Design review of the part built by this model. Coordinates are the model's own, in mm. Face numbers are marked on the shaded views. A direction names the side the tool comes from. Round coordinates to 2 decimals unless told otherwise and drop trailing zeros. Order: outer loops, then holes, each group sorted by start corner. A loop starts at its lowest first (then second) coordinate and runs counter-clockwise, first axis right, second up. Notation, with made-up numbers: (-29.5, 49) - (-17.5, 49) arc R19 cw to (-17.5, 86) - close; hole circle Ø4 at (-5, 51). An arc over 180 degrees is marked (long way). Use CSV: the item, a comma, the result in double quotes.
from build123d import *
from OCP.BRepFilletAPI import BRepFilletAPI_MakeChamfer

# Parameters (mm, degrees)
SKETCH1_W          = 20.2
SKETCH1_H          = 40.2
EXTRUDE1_DEPTH     = 25.4
SKETCH2_W          = 20.2
SKETCH2_H          = 40.2
EXTRUDE2_DEPTH     = 2.38125
SKETCH3_W          = 20.2
SKETCH3_H          = 40.2
EXTRUDE3_DEPTH     = 4.445
EXTRUDE4_DEPTH     = 2.38125
SKETCH5_R          = 7.62
EXTRUDE5_DEPTH     = 3.4925
SKETCH7_W          = 3.5
SKETCH7_H          = 1
EXTRUDE6_DEPTH     = 0.635
SKETCH8_R          = 2.778125
EXTRUDE7_DEPTH     = 3.175
CHAMFER2_SIZE      = 2.54
CHAMFER2_SIZE2     = 1.466469684
FILLET1_R          = 1.016
FILLET2_R          = 1.524
SKETCH9_W          = 6.35
SKETCH9_H          = 2.54
EXTRUDE8_DEPTH     = 2.38125
SKETCH10_W         = 5.08
SKETCH10_H         = 1.27
CUT_EXTRUDE1_DEPTH = 2.38125
CHAMFER3_SIZE      = 0.3
SKETCH11_R         = 3.778125
CUT_EXTRUDE2_DEPTH = 3.175
SKETCH12_R         = 1.15
CUT_EXTRUDE3_DEPTH = 3
CUT_EXTRUDE4_START = -1.5
SKETCH13_R         = 7.62
SKETCH13_R_2       = 5
CUT_EXTRUDE4_DEPTH = 1.5


with BuildPart() as part:
    # Sketch1 → Extrude1 (new body)
    with BuildSketch(Plane(origin=(0, 0, 0), x_dir=(1, 0, 0), z_dir=(0, 1, 0))):
        with Locations((0, -9.94)):
            Rectangle(SKETCH1_W, SKETCH1_H)
    extrude(amount=EXTRUDE1_DEPTH)

    # Sketch2 → Extrude2 (add)
    with BuildSketch(Plane(origin=(0, 25.4, 0), x_dir=(-1, 0, 0), z_dir=(0, 1, 0))):
        with Locations((0, 9.94)):
            Rectangle(SKETCH2_W, SKETCH2_H)
        with BuildLine():
            ThreePointArc((6.731, -15.51418631), (5.08, -11.7094), (3.429, -15.51418631))
            Line((3.429, -15.51418631), (3.429, -16.4846))
            Line((3.429, -16.4846), (-3.429, -16.4846))
            Line((-3.429, -16.4846), (-3.429, -15.51418631))
            ThreePointArc((-3.429, -15.51418631), (-5.08, -11.7094), (-6.731, -15.51418631))
            Line((-6.731, -15.51418631), (-6.731, -16.4846))
            Line((-6.731, -16.4846), (-10.1, -16.4846))
            Line((-10.1, -16.4846), (-10.1, -10.16))
            Line((-10.1, -10.16), (10.1, -10.16))
            Line((10.1, -10.16), (10.1, -16.4846))
            Line((10.1, -16.4846), (6.731, -16.4846))
            Line((6.731, -16.4846), (6.731, -15.51418631))
        make_face()
        with BuildLine():
            ThreePointArc((-6.731, 35.83418631), (-5.08, 32.0294), (-3.429, 35.83418631))
            Line((-3.429, 35.83418631), (-3.429, 36.3646))
            Line((-3.429, 36.3646), (3.429, 36.3646))
            Line((3.429, 36.3646), (3.429, 35.83418631))
            ThreePointArc((3.429, 35.83418631), (5.08, 32.0294), (6.731, 35.83418631))
            Line((6.731, 35.83418631), (6.731, 36.3646))
            Line((6.731, 36.3646), (10.1, 36.3646))
            Line((10.1, 36.3646), (10.1, 30.04))
            Line((10.1, 30.04), (-10.1, 30.04))
            Line((-10.1, 30.04), (-10.1, 36.3646))
            Line((-10.1, 36.3646), (-6.731, 36.3646))
            Line((-6.731, 36.3646), (-6.731, 35.83418631))
        make_face()
    extrude(amount=EXTRUDE2_DEPTH)

    # Sketch3 → Extrude3 (add)
    with BuildSketch(Plane(origin=(0, 27.78125, 0), x_dir=(-1, 0, 0), z_dir=(0, 1, 0))):
        with Locations((0, 9.94)):
            Rectangle(SKETCH3_W, SKETCH3_H)
    extrude(amount=EXTRUDE3_DEPTH)

    # Sketch4 → Extrude4 (add)
    with BuildSketch(Plane(origin=(0, 32.22625, 0), x_dir=(-1, 0, 0), z_dir=(0, 1, 0))):
        with BuildLine():
            Line((9.652, 2.228840954), (9.652, 23.69))
            Line((9.652, 23.69), (4.655896906, 23.69))
            ThreePointArc((4.655896906, 23.69), (0, 26.738), (-4.655896906, 23.69))
            Line((-4.655896906, 23.69), (-9.652, 23.69))
            Line((-9.652, 23.69), (-9.652, 2.228840954))
            ThreePointArc((-9.652, 2.228840954), (0, -9.906), (9.652, 2.228840954))
        make_face()
    extrude(amount=EXTRUDE4_DEPTH)

    # Sketch5 → Extrude5 (add)
    with BuildSketch(Plane(origin=(0, 34.6075, 0), x_dir=(-1, 0, 0), z_dir=(0, 1, 0))):
        with Locations(Location((0, 0, 0), (0, 0, 270))):
            Circle(SKETCH5_R)
    extrude(amount=EXTRUDE5_DEPTH)

    # Sketch7 → Extrude6 (add, symmetric)
    with BuildSketch(Plane(origin=(0, 0, 0), x_dir=(0, 0, -1), z_dir=(1, 0, 0))):
        with Locations((11.91, 28.28125)):
            Rectangle(SKETCH7_W, SKETCH7_H)
    extrude6 = extrude(amount=EXTRUDE6_DEPTH, both=True)

    # Mirror1: Extrude6 across plane
    add(extrude6.mirror(Plane.XY.offset(9.72)))

    # Sketch8 → Extrude7 (add)
    with BuildSketch(Plane(origin=(0, 38.1, 0), x_dir=(-1, 0, 0), z_dir=(0, 1, 0))):
        with Locations(Location((0, 0, 0), (0, 0, 270))):
            Circle(SKETCH8_R)
    extrude(amount=EXTRUDE7_DEPTH)

    # Chamfer2: one chamfer whose edges measure the first distance from different faces: ONE call of the kernel's chamfer builder (chamfer() names one face for all edges)
    chamfer2_edges_1 = [part.edges().sort_by_distance(p)[0] for p in [
        (0, 0, -10.16),
    ]]
    chamfer2_side_1 = [part.faces().sort_by_distance(p)[0] for p in [
        (0, 12.7, -10.16),
    ]]
    chamfer2_edges_2 = [part.edges().sort_by_distance(p)[0] for p in [
        (0, 0, 30.04),
    ]]
    chamfer2_side_2 = [part.faces().sort_by_distance(p)[0] for p in [
        (0, 12.7, 30.04),
    ]]
    chamfer2 = BRepFilletAPI_MakeChamfer(part.part.solid().wrapped)
    for e in chamfer2_edges_1:
        chamfer2.Add(CHAMFER2_SIZE, CHAMFER2_SIZE2, e.wrapped, chamfer2_side_1[0].wrapped)  # the first distance lies on this face
    for e in chamfer2_edges_2:
        chamfer2.Add(CHAMFER2_SIZE, CHAMFER2_SIZE2, e.wrapped, chamfer2_side_2[0].wrapped)  # the first distance lies on this face
    add(Compound.cast(chamfer2.Shape()), mode=Mode.REPLACE)

    # Fillet1
    fillet1_edges = [part.edges().sort_by_distance(p)[0] for p in [
        (-10.1, 30.00375, -10.16),
        (10.1, 30.00375, -10.16),
        (10.1, 30.00375, 30.04),
        (10.1, 0, 9.94),
        (10.1, 1.27, -9.426765158),
        (10.1, 13.97, -10.16),
        (0, 0, -8.693530316),
        (0, 2.54, -10.16),
        (-10.1, 13.97, -10.16),
        (-10.1, 1.27, -9.426765158),
        (10.1, 13.97, 30.04),
        (10.1, 1.27, 29.306765158),
        (0, 2.54, 30.04),
        (-10.1, 0, 9.94),
        (0, 0, 28.573530316),
        (-10.1, 1.27, 29.306765158),
        (-10.1, 13.97, 30.04),
        (-10.1, 30.00375, 30.04),
    ]]
    fillet(fillet1_edges, radius=FILLET1_R)

    # Fillet2
    fillet2_edges = [part.edges().sort_by_distance(p)[0] for p in [
        (-10.1, 26.590625, 36.3646),
        (10.1, 26.590625, 36.3646),
        (-10.1, 26.590625, -16.4846),
        (10.1, 26.590625, -16.4846),
    ]]
    fillet(fillet2_edges, radius=FILLET2_R)

    # Sketch9 → Extrude8 (add)
    with BuildSketch(Plane(origin=(0, 0, -10.16), x_dir=(-1, 0, 0), z_dir=(0, 0, -1))):
        with Locations((0, 4.318)):
            Rectangle(SKETCH9_W, SKETCH9_H)
    extrude(amount=EXTRUDE8_DEPTH)

    # Sketch10 → Cut-Extrude1 (cut)
    with BuildSketch(Plane(origin=(0, 0, -12.54125), x_dir=(-1, 0, 0), z_dir=(0, 0, -1))):
        with Locations((0, 4.318)):
            Rectangle(SKETCH10_W, SKETCH10_H)
    extrude(amount=-CUT_EXTRUDE1_DEPTH, mode=Mode.SUBTRACT)

    # Chamfer3
    chamfer3_edges = [part.edges().sort_by_distance(p)[0] for p in [
        (0, 41.275, 2.778125),
    ]]
    chamfer(chamfer3_edges, length=CHAMFER3_SIZE)

    # Sketch11 → Cut-Extrude2 (cut)
    with BuildSketch(Plane(origin=(0, 41.275, 0), x_dir=(1, 0, 0), z_dir=(0, 1, 0))):
        Circle(SKETCH11_R)
        Polygon((0, -2.778125), (-0.336512839, -2.556068783), (-0.71903166, -2.683462686), (-0.986605724, -2.38187692), (-1.3890625, -2.405926825), (-1.569463059, -2.04536408), (-1.964431026, -1.964431026), (-2.04536408, -1.569463059), (-2.405926825, -1.3890625), (-2.38187692, -0.986605724), (-2.683462686, -0.71903166), (-2.556068783, -0.336512839), (-2.778125, 0), (-2.556068783, 0.336512839), (-2.683462686, 0.71903166), (-2.38187692, 0.986605724), (-2.405926825, 1.3890625), (-2.04536408, 1.569463059), (-1.964431026, 1.964431026), (-1.569463059, 2.04536408), (-1.3890625, 2.405926825), (-0.986605724, 2.38187692), (-0.71903166, 2.683462686), (-0.336512839, 2.556068783), (0, 2.778125), (0.336512839, 2.556068783), (0.71903166, 2.683462686), (0.986605724, 2.38187692), (1.3890625, 2.405926825), (1.569463059, 2.04536408), (1.964431026, 1.964431026), (2.04536408, 1.569463059), (2.405926825, 1.3890625), (2.38187692, 0.986605724), (2.683462686, 0.71903166), (2.556068783, 0.336512839), (2.778125, 0), (2.556068783, -0.336512839), (2.683462686, -0.71903166), (2.38187692, -0.986605724), (2.405926825, -1.3890625), (2.04536408, -1.569463059), (1.964431026, -1.964431026), (1.569463059, -2.04536408), (1.3890625, -2.405926825), (0.986605724, -2.38187692), (0.71903166, -2.683462686), (0.336512839, -2.556068783), align=None, mode=Mode.SUBTRACT)
    extrude(amount=-CUT_EXTRUDE2_DEPTH, mode=Mode.SUBTRACT)

    # Sketch12 → Cut-Extrude3 (cut)
    with BuildSketch(Plane(origin=(0, 41.275, 0), x_dir=(1, 0, 0), z_dir=(0, 1, 0))):
        with Locations(Location((0, 0, 0), (0, 0, 270))):
            Circle(SKETCH12_R)
    extrude(amount=-CUT_EXTRUDE3_DEPTH, mode=Mode.SUBTRACT)

    # Sketch13 → Cut-Extrude4 (cut)
    with BuildSketch(Plane(origin=(0, 38.1, 0), x_dir=(1, 0, 0), z_dir=(0, 1, 0)).offset(CUT_EXTRUDE4_START)):
        with Locations(Location((0, 0, 0), (0, 0, 90))):
            Circle(SKETCH13_R)
        with Locations(Location((0, 0, 0), (0, 0, 270))):
            Circle(SKETCH13_R_2, mode=Mode.SUBTRACT)
    extrude(amount=CUT_EXTRUDE4_DEPTH, mode=Mode.SUBTRACT)


solid = part.part
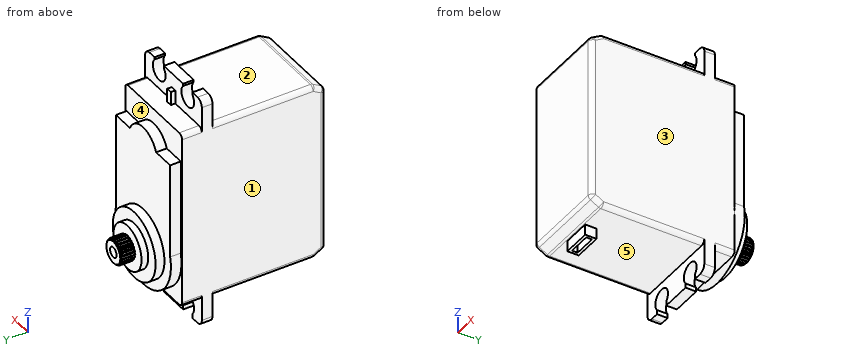
1) We need section D-D (y = 34). Give the boundary of the cut face in (x, z), then the cut area to 3 significant figures.
Data:
outline,"(-9.65, 2.23) arc R9.91 ccw (long way) to (9.65, 2.23) - (9.65, 23.69) - (4.66, 23.69) arc R5.08 ccw to (-4.66, 23.69) - (-9.65, 23.69) - close"
area,"633 mm2"
2) The part is to be moulded in two halves that separate along Y. For the marked faces 3, 4 and 5, say which applies: +Y half, -Y half, draft (parallel to the pull), parting line (faces both ways), or undercut.
Data:
face 3,"draft"
face 4,"+Y half"
face 5,"undercut"
3) We need section B-B (y = 26.5). Give the boundary of the cut face in (x, z).
Data:
outline,"(-10.1, -14.96) arc R1.52 ccw to (-8.58, -16.48) - (-6.73, -16.48) - (-6.73, -15.51) arc R2.26 cw (long way) to (-3.43, -15.51) - (-3.43, -16.48) - (3.43, -16.48) - (3.43, -15.51) arc R2.26 cw (long way) to (6.73, -15.51) - (6.73, -16.48) - (8.58, -16.48) arc R1.52 ccw to (10.1, -14.96) - (10.1, 34.84) arc R1.52 ccw to (8.58, 36.36) - (6.73, 36.36) - (6.73, 35.83) arc R2.26 cw (long way) to (3.43, 35.83) - (3.43, 36.36) - (-3.43, 36.36) - (-3.43, 35.83) arc R2.26 cw (long way) to (-6.73, 35.83) - (-6.73, 36.36) - (-8.58, 36.36) arc R1.52 ccw to (-10.1, 34.84) - close"
4) To check wall thickness, follow L1, parallel to X at y = 26.1, z = 34.29; L2, parallel to Y at x = -0.5, z = -10.5; L3, parallel to Z at x = -6, y = 28.5. State the ranges of each line that lie inside material, in increasing order. Write a range as from..to.
Data:
L1,"x = -10.1..-7.34, -2.82..2.82, 7.34..10.1"
L2,"y = 3.05..3.68, 4.95..5.59, 25.4..28.78"
L3,"z = -10.16..30.04"
5) Insertion check: pin 1 Ø2.5 at (y, z) = (34, 9.5) entering from -X; pin 2 Ø2 at (x, y) = (-4, 21) entering from +Z; pin 3 Ø1 at (x, y) = (5, 26.5) entering from -Z. Each pin has a flat end and moves straight along its axis. Give the tip position at first contact, or say it passes through.
Data:
pin 1,"stops at x = -9.65"
pin 2,"stops at z = 30.04"
pin 3,"stops at z = -11.79"
6) We need section A-A (z = 19). Give the boundary of the cut face in (x, y).
Data:
outline,"(-10.1, 1.02) arc R1.02 ccw to (-9.08, 0) - (9.08, 0) arc R1.02 ccw to (10.1, 1.02) - (10.1, 32.23) - (9.65, 32.23) - (9.65, 34.61) - (-9.65, 34.61) - (-9.65, 32.23) - (-10.1, 32.23) - close"
7) For the marked faces 1 and 2, list the 3-axis set-ups (+Z, -Z, +X, -X, +Y, -Y) from which the entire face can be reached by the end or side of a thin tool; tool diameter is ignored.
Data:
face 1,"+Z, -Z, -X, +Y, -Y"
face 2,"+Z, +X, -X, -Y"
8) We need section C-C (y = 13). Give the boundary of the cut face in (x, z).
Data:
outline,"(-10.1, -9.14) arc R1.02 ccw to (-9.08, -10.16) - (9.08, -10.16) arc R1.02 ccw to (10.1, -9.14) - (10.1, 29.02) arc R1.02 ccw to (9.08, 30.04) - (-9.08, 30.04) arc R1.02 ccw to (-10.1, 29.02) - close"
